Model file for the job. Use its own axes, mm. Face numbers are marked on the shaded views. A direction names the side the tool comes from. Coordinates: 2 decimals unless noted, no trailing zeros. Write each loop counter-clockwise with the first axis right and the second up, starting at its lowest first coordinate (ties: lowest second). Pieces come first, ordered by that corner, then holes. Notation, with made-up numbers: (49.25, -12.75) - (106.25, -12.75) arc R11 ccw to (106.25, 0.25) - close; hole circle Ø9 at (-40, 66). An arc over 180 degrees is marked (long way). Put each result on its own line as item: value. Start each with the question number.
1. Which spindle directions (+Z, -Z, +X, -X, +Y, -Y) get a long thin tool onto all of the face, cutting with end or side? Do the marked faces 4 and 5. Say none if no direction does.
2. Pull direction Z, two halves, no side cores. Call the marked faces 1, 2 and 3: released by +Z, released by -Z, zero draft, split by the parting line, or undercut.
3. Saw through at B-B, the plane x = 0. Write the cut outline in (y, z).
4. Saw through at A-A, the plane z = 0. Write the cut outline in (x, y).
5. Saw through at C-C, the plane y = 4.25. Write the cut outline in (x, z), plus the area to 3 significant figures.
6. Saw through at D-D, the plane y = 7.25. Write the cut outline in (x, z), plus the area to 3 significant figures.
7. Drill centre lines: L1, parallel to Z at x = 0, y = 3.6; L2, parallel to X at y = 3.8, z = 8.75; L3, parallel to X at y = 1.3, z = 8.75. Where is each one in solid material? Low to high. Write a range as from..to.
8. Drop flat-ended pins along their axis: P1, Ø6, axis at x = 1.5, y = 6, coming from the -Z side; P2, Ø1, axis at x = 18.5, y = 2.5, coming from the +Z side; P3, Ø2, axis at y = 4.5, z = 11, coming from the -X side. Give the stop position or say it passes through.
```python
from build123d import *

# Parameters (mm, degrees)
SKETCH1_R               = 26
BOSS_EXTRUDE1_DEPTH     = 5
SKETCH1_3_R             = 3
CUT_EXTRUDE1_DEPTH      = 6
CUT_EXTRUDE1_DEPTH_BACK = 1
SKETCH1_4_R             = 12.5
BOSS_EXTRUDE2_DEPTH     = 12
SKETCH1_5_R             = 8
CUT_EXTRUDE2_DEPTH      = 13
CUT_EXTRUDE2_DEPTH_BACK = 1
FILLET1_R               = 2


with BuildPart() as part:
    # Sketch1 → Boss-Extrude1 (new body)
    with BuildSketch(Plane(origin=(0, 0, 0), x_dir=(1, 0, 0), z_dir=(0, 1, 0))):
        Circle(SKETCH1_R)
    extrude(amount=BOSS_EXTRUDE1_DEPTH)

    # Sketch1<3> → Cut-Extrude1 (cut, two sides)
    with BuildSketch(Plane(origin=(0, 0, 0), x_dir=(1, 0, 0), z_dir=(0, 1, 0))) as cut_extrude1_sk:
        with Locations((0, 17.5)):
            Circle(SKETCH1_3_R)
        with Locations((15.155444566, -8.75)):
            Circle(SKETCH1_3_R)
        with Locations((-15.155444566, -8.75)):
            Circle(SKETCH1_3_R)
    extrude(amount=CUT_EXTRUDE1_DEPTH, mode=Mode.SUBTRACT)
    extrude(cut_extrude1_sk.sketch, amount=-CUT_EXTRUDE1_DEPTH_BACK, mode=Mode.SUBTRACT)

    # Sketch1<4> → Boss-Extrude2 (add)
    with BuildSketch(Plane(origin=(0, 0, 0), x_dir=(1, 0, 0), z_dir=(0, 1, 0))):
        Circle(SKETCH1_4_R)
    extrude(amount=BOSS_EXTRUDE2_DEPTH)

    # Sketch1<5> → Cut-Extrude2 (cut, two sides)
    with BuildSketch(Plane(origin=(0, 0, 0), x_dir=(1, 0, 0), z_dir=(0, 1, 0))) as cut_extrude2_sk:
        Circle(SKETCH1_5_R)
    extrude(amount=CUT_EXTRUDE2_DEPTH, mode=Mode.SUBTRACT)
    extrude(cut_extrude2_sk.sketch, amount=-CUT_EXTRUDE2_DEPTH_BACK, mode=Mode.SUBTRACT)

    # Fillet1
    fillet1_edges = [part.edges().sort_by_distance(p)[0] for p in [
        (-26, 0, 0),
    ]]
    fillet(fillet1_edges, radius=FILLET1_R)


solid = part.part
```
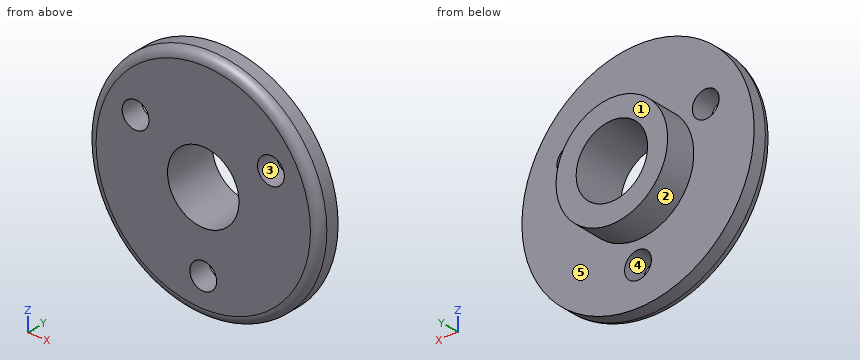
Final values:
1. face 4: +Y, -Y
1. face 5: +Y
2. face 1: zero draft
2. face 2: split by the parting line
2. face 3: undercut
3. outline: (0, -24) arc R2 ccw to (2, -26) - (5, -26) - (5, -20.5) - (0, -20.5) - close; (0, -14.5) - (5, -14.5) - (5, -12.5) - (12, -12.5) - (12, -8) - (0, -8) - close; (0, 8) - (12, 8) - (12, 12.5) - (5, 12.5) - (5, 26) - (2, 26) arc R2 ccw to (0, 24) - close
4. outline: (-26, 2) arc R2 ccw to (-24, 0) - (-8, 0) - (-8, 12) - (-12.5, 12) - (-12.5, 5) - (-26, 5) - close; (8, 0) - (24, 0) arc R2 ccw to (26, 2) - (26, 5) - (12.5, 5) - (12.5, 12) - (8, 12) - close
5. outline: circle Ø52 at (0, 0); hole circle Ø6 at (-15.16, 8.75); hole circle Ø16 at (0, 0); hole circle Ø6 at (0, -17.5); hole circle Ø6 at (15.16, 8.75)
5. area: 1,840 mm²
6. outline: circle Ø25 at (0, 0); hole circle Ø16 at (0, 0)
6. area: 290 mm²
7. L1: z = -26..-20.5, -14.5..-8, 8..26
7. L2: x = -24.48..-18.16, -12.16..12.16, 18.16..24.48
7. L3: x = -24.35..-18.16, -12.16..12.16, 18.16..24.35
8. P1: stops at z = -26
8. P2: stops at z = 18.76
8. P3: stops at x = -24
